Check sheet for the drawn part. Datum: minimum x, y, z corner. Units: mm. A direction names the side the tool comes from. Give positions to 0.01 mm unless a question says otherwise; leave off trailing zeros. Loops run counter-clockwise (first coordinate to the right, second up) from the corner with the lowest first, then second, coordinate; pieces in that order, holes last. Notation, with made-up numbers: (-0.5, 44.5) - (43.5, 44.5) arc R26 cw to (43.5, 83.5) - close; hole circle Ø3 at (-22, -29). An arc over 180 degrees is marked (long way). One line per item, written item: value. Start each with the question number.
1. Sectioned sample at D-D (x = 12.7). Record the cut outline in (y, z).
2. Access from +Z, -Z, +X, -X, +Y, -Y to the whole of each face (thin tool, end or side, straight path). Record for the marked faces 5, 6 and 7.
3. Sectioned sample at B-B (z = 14.5). Record the cut outline in (x, y), plus the area to 3 significant figures.
4. Sectioned sample at C-C (y = 3.5). Record the cut outline in (x, z), plus the area to 3 significant figures.
5. Mould release check, pull along Z, two halves, no side actions. Record for the marked faces 1, 2, 3 and 4: pulls with the +Z half, pulls with the -Z half, needs draft (parallel to the pull), parting line crosses it, or undercut.
6. Gauge pin test, flat ends, axial feed: pin 1 (6 mm diameter, centred on y = 3.5, z = 68.5, fed in from +X); pin 2 (3 mm diameter, centred on y = 23.5, z = 100, fed in from -X). Record the tip position at first contact, or that the pin passes through.
7. Sectioned sample at A-A (x = 107.5). Record the cut outline in (y, z).
8. Scan lines: L1, parallel to X at y = 12.7, z = 13.25; L2, parallel to Y at x = 50, z = 82; L3, parallel to X at y = 3.5, z = 30. Record each from-to range of solid material in increasing order. Write a range as [from, to].
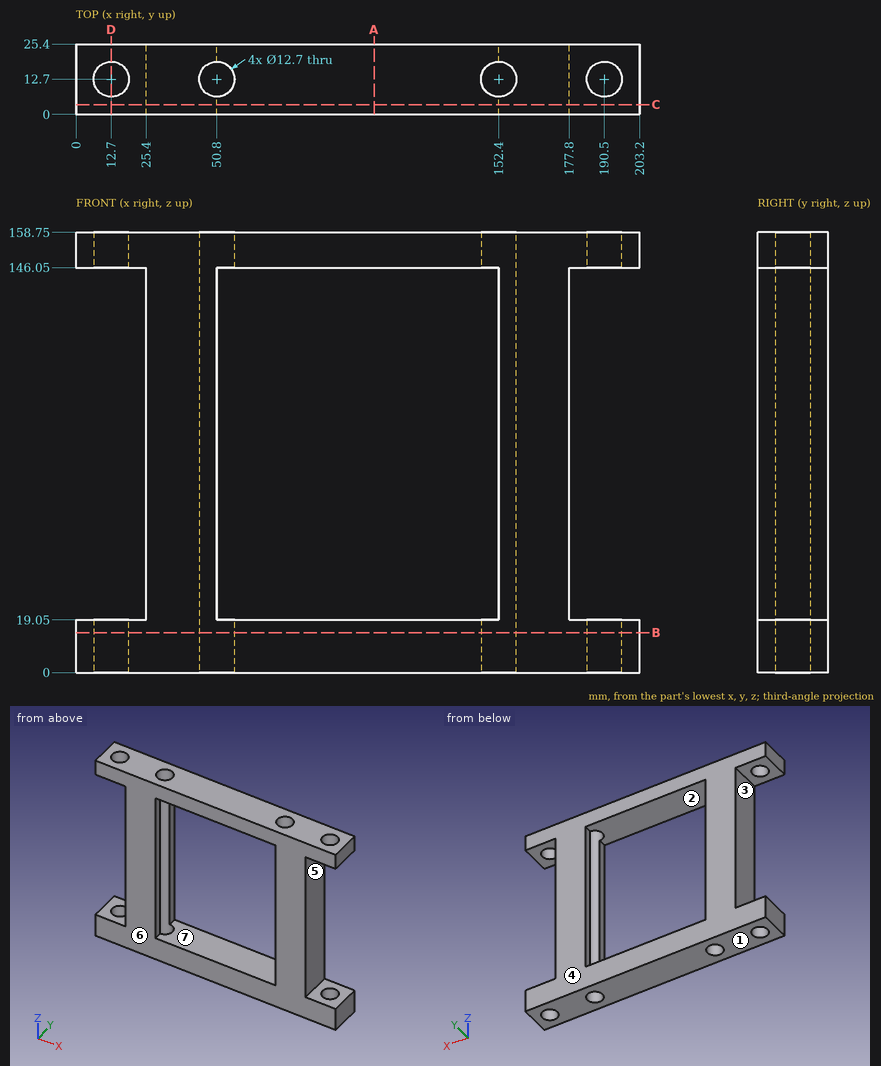
Results are:
1. outline: (0, 0) - (6.35, 0) - (6.35, 19.05) - (0, 19.05) - close; (0, 146.05) - (6.35, 146.05) - (6.35, 158.75) - (0, 158.75) - close; (19.05, 0) - (25.4, 0) - (25.4, 19.05) - (19.05, 19.05) - close; (19.05, 146.05) - (25.4, 146.05) - (25.4, 158.75) - (19.05, 158.75) - close
2. face 5: +X, +Y, -Y
2. face 6: +Z, -Z, +X, -X, -Y
2. face 7: +Y, -Y
3. outline: (0, 0) - (203.2, 0) - (203.2, 25.4) - (0, 25.4) - close; hole circle Ø12.7 at (12.7, 12.7); hole circle Ø12.7 at (50.8, 12.7); hole circle Ø12.7 at (152.4, 12.7); hole circle Ø12.7 at (190.5, 12.7)
3. area: 4,650 mm^2
4. outline: (0, 0) - (203.2, 0) - (203.2, 19.05) - (177.8, 19.05) - (177.8, 146.05) - (203.2, 146.05) - (203.2, 158.75) - (0, 158.75) - (0, 146.05) - (25.4, 146.05) - (25.4, 19.05) - (0, 19.05) - close; hole (50.8, 19.05) - (152.4, 19.05) - (152.4, 146.05) - (50.8, 146.05) - close
4. area: 12,900 mm^2
5. face 1: pulls with the -Z half
5. face 2: undercut
5. face 3: undercut
5. face 4: needs draft
6. pin 1: stops at x = 177.8
6. pin 2: stops at x = 25.4
7. outline: (0, 0) - (25.4, 0) - (25.4, 19.05) - (0, 19.05) - close; (0, 146.05) - (25.4, 146.05) - (25.4, 158.75) - (0, 158.75) - close
8. L1: x = [0, 6.35], [19.05, 44.45], [57.15, 146.05], [158.75, 184.15], [196.85, 203.2]
8. L2: y = [0, 6.4], [19, 25.4]
8. L3: x = [25.4, 50.8], [152.4, 177.8]
